For this review, use the dimensioned drawing (mm, ordinates from the lowest corner) and the shaded views. A direction names the side the tool comes from. Round coordinates to 2 decimals unless told otherwise and drop trailing zeros. Order: outer loops, then holes, each group sorted by start corner. A loop starts at its lowest first (then second) coordinate and runs counter-clockwise, first axis right, second up. Notation, with made-up numbers: (74.5, -13) -> (110.5, -13) arc R26 cw to (110.5, 3) -> close; hole circle Ø1 at (36.25, 34). An arc over 180 degrees is marked (long way). Answer in a Markdown table with one row per item.
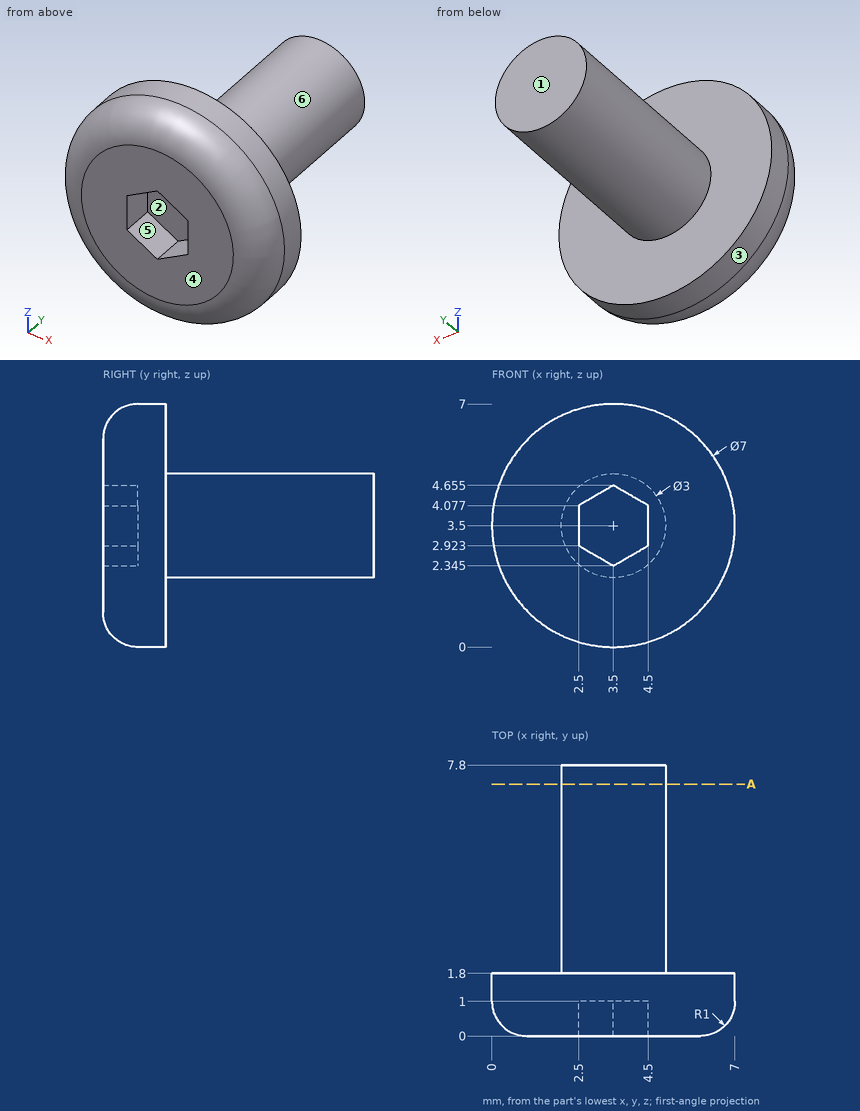
Q1. The part is to be moulded in two halves that separate along Z. For the marked faces 1, 2 and 3, say which applies: +Z half, -Z half, draft (parallel to the pull), parting line (faces both ways), or undercut.
Answer key:
| item | result |
|---|---|
| face 1 | draft |
| face 2 | undercut |
| face 3 | parting line |
Q2. Clearance check with flat-ended pins moving along their axes: pin 1 Ø4 at (x, y) = (5.5, 6.5) entering from -Z; pin 2 Ø1.5 at (y, z) = (3, 5.5) entering from -X; pin 3 Ø1.6 at (x, z) = (3.5, 3.5) entering from -Y. State where each tip first meets the part, or that it passes through.
Answer key:
| item | result |
|---|---|
| pin 1 | stops at z = 2 |
| pin 2 | stops at x = 2.67 |
| pin 3 | stops at y = 1 |
Q3. To check wall thickness, follow probe 1 along Y at (x, z) = (1.75, 2.5); probe 2 along X at (y, z) = (5, 3.5); probe 3 along X at (y, z) = (6, 4.5). State the ranges of each line that lie inside material, in increasing order.
Answer key:
| item | result |
|---|---|
| probe 1 | y = 0 to 1.8 |
| probe 2 | x = 2 to 5 |
| probe 3 | x = 2.38 to 4.62 |
Q4. Tool access review of the marked faces 4, 5 and 6: name each direction out of +Z, -Z, +X, -X, +Y, -Y from which nothing blocks a thin tool from reaching the whole face with its end or side.
Answer key:
| item | result |
|---|---|
| face 4 | +Z, -Z, +X, -X, -Y |
| face 5 | -Y |
| face 6 | +Y |
Q5. Take a section at A-A, the plane y = 7.25. Write out the cut boundary in (x, z).
Answer key:
| item | result |
|---|---|
| outline | circle Ø3 at (3.5, 3.5) |
